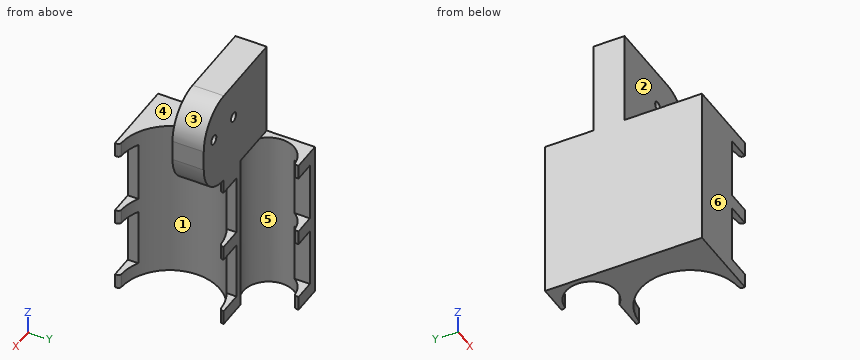
from build123d import *

# Parameters (mm, degrees)
BOSS_EXTRUDE1_DEPTH = 70
SKETCH2_W           = 30.127897987
SKETCH2_H           = 25.625
CUT_EXTRUDE1_DEPTH  = 10
SKETCH3_W           = 36.135462637
SKETCH3_H           = 24.960917338
SKETCH3_H_2         = 26.289082662
CUT_EXTRUDE2_DEPTH  = 88.210896549
SKETCH5_W           = 40.769231001
SKETCH5_H           = 13.5
BOSS_EXTRUDE2_DEPTH = 50
SKETCH6_R           = 2
CUT_EXTRUDE3_DEPTH  = 50
FILLET1_R           = 1.25
FILLET2_R           = 16


with BuildPart() as part:
    # Sketch1 → Boss-Extrude1 (new body)
    with BuildSketch(Plane.XY):
        with BuildLine():
            Line((22.473811518, 84.75800041), (22.473811518, 83.058719541))
            ThreePointArc((22.473811518, 83.058719541), (0.883811518, 61.468719541), (22.473811518, 39.878719541))
            Line((22.473811518, 39.878719541), (22.473811518, 37.846719541))
            Line((22.473811518, 37.846719541), (-11.673355367, 37.846719541))
            Line((-11.673355367, 37.846719541), (-11.673355367, 105.594024014))
            Line((-11.673355367, 105.594024014), (1.358644633, 105.594024014))
            Line((1.358644633, 105.594024014), (1.358644633, 103.665116534))
            ThreePointArc((1.358644633, 103.665116534), (-8.83886186, 88.540693991), (9.005703845, 84.75800041))
            Line((9.005703845, 84.75800041), (22.473811518, 84.75800041))
        make_face()
    extrude(amount=-BOSS_EXTRUDE1_DEPTH)

    # Sketch2 → Cut-Extrude1 (cut)
    with BuildSketch(Plane(origin=(0, 105.594024014, 0), x_dir=(1, 0, 0), z_dir=(0, 1, 0))):
        with Locations((7.409862525, 50.9375)):
            Rectangle(SKETCH2_W, SKETCH2_H)
        with Locations((7.409862525, 19.0625)):
            Rectangle(SKETCH2_W, SKETCH2_H)
    extrude(amount=-CUT_EXTRUDE1_DEPTH, mode=Mode.SUBTRACT)

    # Sketch3 → Cut-Extrude2 (cut, through all)
    with BuildSketch(Plane(origin=(0, 84.75800041, 0), x_dir=(1, 0, 0), z_dir=(0, 1, 0))):
        with Locations((30.426375951, 51.269541331)):
            Rectangle(SKETCH3_W, SKETCH3_H)
        with Locations((30.426375951, 19.394541331)):
            Rectangle(SKETCH3_W, SKETCH3_H_2)
    extrude(amount=-CUT_EXTRUDE2_DEPTH, mode=Mode.SUBTRACT)

    # Sketch5 → Boss-Extrude2 (add)
    with BuildSketch(Plane.ZY.offset(11.673355367)):
        with Locations((20.384615501, 78.00800041)):
            Rectangle(SKETCH5_W, SKETCH5_H)
    extrude(amount=-BOSS_EXTRUDE2_DEPTH)

    # Sketch6 → Cut-Extrude3 (cut)
    with BuildSketch(Plane(origin=(0, 84.75800041, 0), x_dir=(1, 0, 0), z_dir=(0, 1, 0))):
        with Locations(Location((14.647627353, -25, 0), (0, 0, 270))):
            Circle(SKETCH6_R)
        with Locations(Location((30.329421103, -25, 0), (0, 0, 270))):
            Circle(SKETCH6_R)
    extrude(amount=-CUT_EXTRUDE3_DEPTH, mode=Mode.SUBTRACT)

    # Fillet1
    fillet1_edges = [part.edges().sort_by_distance(p)[0] for p in [
        (1.358644633, 103.665116534, -66.875),
        (22.473811518, 83.058719541, -66.875),
        (22.473811518, 39.878719541, -66.875),
        (1.358644633, 103.665116534, -35),
        (1.358644633, 103.665116534, -3.125),
        (22.473811518, 39.878719541, -35.664082662),
        (22.473811518, 39.878719541, -3.125),
        (22.473811518, 83.058719541, -35.664082662),
        (22.473811518, 83.058719541, -3.125),
    ]]
    fillet(fillet1_edges, radius=FILLET1_R)

    # Fillet2
    fillet2_edges = [part.edges().sort_by_distance(p)[0] for p in [
        (38.326644633, 78.00800041, 0),
        (38.326644633, 78.00800041, 40.769231001),
    ]]
    fillet(fillet2_edges, radius=FILLET2_R)


solid = part.part
Design review of the part built by this model. Coordinates are the model's own, in mm. Face numbers are marked on the shaded views. A direction names the side the tool comes from. Round coordinates to 2 decimals unless told otherwise and drop trailing zeros. Order: outer loops, then holes, each group sorted by start corner. A loop starts at its lowest first (then second) coordinate and runs counter-clockwise, first axis right, second up. Notation, with made-up numbers: M 7,51 L 49,51 A19 cw 49,77 Z; hole C 45,-20 d7. An arc over 180 degrees is marked long. Answer as CSV lines item,"result". Start each with the question number.
1) The part is to be moulded in two halves that separate along Y. For the marked faces 4, 5 and 6, say which applies: +Y half, -Y half, draft (parallel to the pull), parting line (faces both ways), or undercut.
2) Tool access review of the marked faces 1, 2 and 3: name each direction out of +Z, -Z, +X, -X, +Y, -Y from which nothing blocks a thin tool from reaching the whole face with its end or side.
3) Wall thickness on line 1 along X through (y, z) = (75.5, 25); line 2 along Z through (x, y) = (22.5, 72); line 3 along Y through (x, z) = (36, 29): over which ranges is each line inside the solid? List them lowest first. Write a range as [from, to].
4) Add section A-A (x = 19.5). Give the boundary of the cut face in (y, z).
5) Add section B-B (z = -35). Give the boundary of the cut face in (x, y).
6) Add section C-C (x = 7). Give the boundary of the cut face in (y, z), then the cut area to 3 significant figures.
7) Add section D-D (y = 76). Give the boundary of the cut face in (x, z), then the cut area to 3 significant figures.
8) For pin 1 Ø1.5 at (x, y) = (25, 79.5) entering from +Z; pin 2 Ø5.5 at (x, y) = (-3.5, 102.5) entering from -Z; pin 3 Ø6.5 at (x, z) = (14.65, 25) entering from +Y; pin 4 Ø10.5 at (x, y) = (-5.5, 98) entering from +Z, all flat-tipped, find the tip position at first contact; note any pin that passes through.
Resolved:
1,face 4,"draft"
1,face 5,"undercut"
1,face 6,"-Y half"
2,face 1,"-Z, +X"
2,face 2,"+Z, +X, -X, -Y"
2,face 3,"+Z, +X, +Y, -Y"
3,line 1,"[-11.67, 12.65], [16.65, 28.33], [32.33, 38.32]"
3,line 2,"[0, 40.77]"
3,line 3,"[71.26, 84.76]"
4,outline,"M 37.85,-70 L 40.08,-70 L 40.08,-63.75 L 37.85,-63.75 Z; M 37.85,-38.79 L 40.08,-38.79 L 40.08,-32.54 L 37.85,-32.54 Z; M 37.85,-6.25 L 40.08,-6.25 L 40.08,0 L 37.85,0 Z; M 71.26,0 L 82.85,0 L 82.85,-6.25 L 84.76,-6.25 L 84.76,40.77 L 71.26,40.77 Z; M 82.85,-70 L 84.76,-70 L 84.76,-63.75 L 82.85,-63.75 Z; M 82.85,-38.79 L 84.76,-38.79 L 84.76,-32.54 L 82.85,-32.54 Z"
5,outline,"M -11.67,37.85 L 22.47,37.85 L 22.47,38.66 A1.25 ccw 21.29,39.91 A21.59 cw 21.29,83.03 A1.25 ccw 22.47,84.27 L 22.47,84.76 L 9.01,84.76 A11 cw long 0.24,103.61 A1.25 ccw 1.36,104.85 L 1.36,105.59 L -11.67,105.59 Z"
6,outline,"M 37.85,-70 L 46.41,-70 L 46.41,0 L 37.85,0 Z; M 71.26,0 L 76.52,0 L 76.52,-70 L 83.22,-70 L 83.22,0 L 84.76,0 L 84.76,40.77 L 71.26,40.77 Z"
6,area,"1,620 mm^2"
7,outline,"M -11.67,-70 L 6.51,-70 L 6.51,0 L 22.33,0 A16 ccw 38.33,16 L 38.33,24.77 A16 ccw 22.33,40.77 L -11.67,40.77 Z; hole C 14.65,25 d4; hole C 30.33,25 d4"
7,area,"3,180 mm^2"
8,pin 1,"z = 40.65"
8,pin 2,"z = -70"
8,pin 3,"y = 84.76"
8,pin 4,"z = 0"
